```python
from build123d import *

# Parameters (mm, degrees)
CROQUIS1_R              = 100
SALIENTE_EXTRUIR1_DEPTH = 3
CROQUIS3_R              = 110
CORTAR_EXTRUIR1_DEPTH   = 3
REDONDEO1_R             = 10
CORTAR_EXTRUIR2_DEPTH   = 10
CORTAR_EXTRUIR3_DEPTH   = 10
CROQUIS8_R              = 1.5
CROQUIS8_R_2            = 1.502317269
CROQUIS8_R_3            = 2
CORTAR_EXTRUIR4_DEPTH   = 10
CROQUIS9_R              = 1.5
CROQUIS9_W              = 4.5
CROQUIS9_H              = 7.5
CROQUIS9_W_2            = 7.5
CROQUIS9_H_2            = 4.5
CORTAR_EXTRUIR5_DEPTH   = 10


with BuildPart() as part:
    # Croquis1 → Saliente-Extruir1 (new body)
    with BuildSketch(Plane.XY):
        Circle(CROQUIS1_R)
    extrude(amount=SALIENTE_EXTRUIR1_DEPTH)

    # Croquis3 → Cortar-Extruir1 (cut)
    with BuildSketch(Plane.XY.offset(3)):
        with Locations((190, 0)):
            Circle(CROQUIS3_R)
    extrude(amount=-CORTAR_EXTRUIR1_DEPTH, mode=Mode.SUBTRACT)

    # Redondeo1
    redondeo1_edges = [part.edges().sort_by_distance(p)[0] for p in [
        (89.473684211, -44.659375654, 1.5),
        (89.473684211, 44.659375654, 1.5),
    ]]
    fillet(redondeo1_edges, radius=REDONDEO1_R)

    # Croquis5 → Cortar-Extruir2 (cut)
    with BuildSketch(Plane.XY.offset(3)):
        Polygon((-29.69848481, -9.899494937), (-9.899494937, -29.69848481), (-64.346717088, -84.145706961), (-84.145706961, -64.346717088), align=None)
        Polygon((-9.899494937, 29.69848481), (-29.69848481, 9.899494937), (-84.145706961, 64.346717088), (-64.346717088, 84.145706961), align=None)
        Polygon((29.69848481, 9.899494937), (9.899494937, 29.69848481), (64.346717088, 84.145706961), (84.145706961, 64.346717088), align=None)
        Polygon((9.899494937, -29.69848481), (29.69848481, -9.899494937), (84.145706961, -64.346717088), (64.346717088, -84.145706961), align=None)
    extrude(amount=-CORTAR_EXTRUIR2_DEPTH, mode=Mode.SUBTRACT)

    # Croquis7 → Cortar-Extruir3 (cut)
    with BuildSketch(Plane.XY.offset(3)):
        Polygon((-71.939339828, -40.119534675), (-40.119534675, -71.939339828), (-57.090097423, -88.909902577), (-88.909902577, -57.090097423), align=None)
        Polygon((-40.119534675, 71.939339828), (-71.939339828, 40.119534675), (-88.909902577, 57.090097423), (-57.090097423, 88.909902577), align=None)
        Polygon((71.939339828, 40.119534675), (40.119534675, 71.939339828), (57.090097423, 88.909902577), (88.909902577, 57.090097423), align=None)
        Polygon((40.119534675, -71.939339828), (71.939339828, -40.119534675), (88.909902577, -57.090097423), (57.090097423, -88.909902577), align=None)
        Polygon((-21.566756826, -18.03122292), (-18.03122292, -21.566756826), (-14.495689014, -18.03122292), (-18.03122292, -14.495689014), align=None)
        Polygon((-21.566756826, 18.03122292), (-18.03122292, 14.495689014), (-14.495689014, 18.03122292), (-18.03122292, 21.566756826), align=None)
        Polygon((18.03122292, 21.566756826), (14.495689014, 18.03122292), (18.03122292, 14.495689014), (21.566756826, 18.03122292), align=None)
        Polygon((21.566756826, -18.03122292), (18.03122292, -14.495689014), (14.495689014, -18.03122292), (18.03122292, -21.566756826), align=None)
    extrude(amount=-CORTAR_EXTRUIR3_DEPTH, mode=Mode.SUBTRACT)

    # Croquis8 → Cortar-Extruir4 (cut)
    with BuildSketch(Plane.XY.offset(3)):
        with Locations((-64.762205999, 40.904423202)):
            Circle(CROQUIS8_R)
        with Locations((-48.852303422, 24.994520625)):
            Circle(CROQUIS8_R_2)
        with Locations((-24.994520625, 48.852303422)):
            Circle(CROQUIS8_R)
        with Locations((-40.904423202, 64.762205999)):
            Circle(CROQUIS8_R)
        with Locations((64.762205999, 40.904423202)):
            Circle(CROQUIS8_R)
        with Locations((48.852303422, 24.994520625)):
            Circle(CROQUIS8_R)
        with Locations((24.994520625, 48.852303422)):
            Circle(CROQUIS8_R_2)
        with Locations((40.904423202, 64.762205999)):
            Circle(CROQUIS8_R)
        with Locations((40.904423202, -64.762205999)):
            Circle(CROQUIS8_R)
        with Locations((24.994520625, -48.852303422)):
            Circle(CROQUIS8_R)
        with Locations((48.852303422, -24.994520625)):
            Circle(CROQUIS8_R_2)
        with Locations((64.762205999, -40.904423202)):
            Circle(CROQUIS8_R)
        with Locations((-64.762205999, -40.904423202)):
            Circle(CROQUIS8_R)
        with Locations((-48.852303422, -24.994520625)):
            Circle(CROQUIS8_R)
        with Locations((-24.994520625, -48.852303422)):
            Circle(CROQUIS8_R_2)
        with Locations((-40.904423202, -64.762205999)):
            Circle(CROQUIS8_R)
        with Locations((0, 92)):
            Circle(CROQUIS8_R_3)
        with Locations((0, -92)):
            Circle(CROQUIS8_R_3)
        with Locations((72, 31.694913472)):
            Circle(CROQUIS8_R_3)
        with Locations((72, -31.694913472)):
            Circle(CROQUIS8_R_3)
        with Locations((-85, -30)):
            Circle(CROQUIS8_R_3)
        with Locations((-85, 30)):
            Circle(CROQUIS8_R_3)
    extrude(amount=-CORTAR_EXTRUIR4_DEPTH, mode=Mode.SUBTRACT)

    # Croquis9 → Cortar-Extruir5 (cut)
    with BuildSketch(Plane.XY.offset(3)):
        with Locations((73.1, -4.5)):
            Circle(CROQUIS9_R)
        with Locations((35.9, 4.5)):
            Circle(CROQUIS9_R)
        with Locations((73.1, 4.5)):
            Circle(CROQUIS9_R)
        with Locations((35.9, -4.5)):
            Circle(CROQUIS9_R)
        with Locations((-91.190074744, 4.5)):
            Circle(CROQUIS9_R)
        with Locations((-91.190074744, -4.5)):
            Circle(CROQUIS9_R)
        with Locations((-53.990074744, 4.5)):
            Circle(CROQUIS9_R)
        with Locations((-53.990074744, -4.5)):
            Circle(CROQUIS9_R)
        with Locations((-4.5, 85)):
            Circle(CROQUIS9_R)
        with Locations((4.5, 85)):
            Circle(CROQUIS9_R)
        with Locations((-4.5, 47.8)):
            Circle(CROQUIS9_R)
        with Locations((4.5, 47.8)):
            Circle(CROQUIS9_R)
        with Locations((-4.5, -47.8)):
            Circle(CROQUIS9_R)
        with Locations((4.5, -47.8)):
            Circle(CROQUIS9_R)
        with Locations((4.5, -85)):
            Circle(CROQUIS9_R)
        with Locations((-4.5, -85)):
            Circle(CROQUIS9_R)
        with Locations((39.85, 0)):
            Rectangle(CROQUIS9_W, CROQUIS9_H)
        with Locations((0, -51.75)):
            Rectangle(CROQUIS9_W_2, CROQUIS9_H_2)
        with Locations((-57.940074744, 0)):
            Rectangle(CROQUIS9_W, CROQUIS9_H)
        with Locations((0, 51.75)):
            Rectangle(CROQUIS9_W_2, CROQUIS9_H_2)
    extrude(amount=-CORTAR_EXTRUIR5_DEPTH, mode=Mode.SUBTRACT)


solid = part.part
```
The model under review builds one solid part; all positions refer to its coordinate system, in mm. A direction names the side the tool comes from. Round coordinates to 2 decimals unless told otherwise and drop trailing zeros. Order: outer loops, then holes, each group sorted by start corner. A loop starts at its lowest first (then second) coordinate and runs counter-clockwise, first axis right, second up. Notation, with made-up numbers: (-2, -37.75) - (5, -37.75) arc R11 cw to (5, -24.75) - close; hole circle Ø10 at (78.5, -2.5). An arc over 180 degrees is marked (long way). Answer in a Markdown table with one row per item.
(1) Machinability: for faces 5 (the face through (-68.89, 43.17, 1.52)), 6 (the face through (-43.08, 68.98, 1.52)), 7 (the face through (25.7, 13.9, 1.5)), 8 (the face through (78.28, -46.46, 1.52)), which of the approach directions +Z, -Z, +X, -X, +Y, -Y give a long, thin tool a straight path to every point of the face, cutting with its end or side? Answer none if there is none.
Result set:
| item | result |
|---|---|
| face 5 | +Z, -Z, +Y |
| face 6 | +Z, -Z, -X |
| face 7 | +Z, -Z |
| face 8 | +Z, -Z, -Y |
(2) Take a section at A-A on z = 1.5. Count the separate pieces of the cut face and the enclosed holes in it, plus the area to 3 significant figures.
Result set:
| item | result |
|---|---|
| separate pieces | 1 |
| enclosed holes | 42 |
| area | 20,300 mm2 |
(3) Take a section at B-B on y = -58.5. Write out the cut boundary in (x, z).
Result set:
| item | result |
|---|---|
| outline | (-38.7, 0) - (38.7, 0) - (38.7, 3) - (-38.7, 3) - close |
(4) For line 1 (Y direction, x = 17, z = 0.35); line 2 (Y direction, x = -12.5, z = 2.65); line 3 (Y direction, x = 27, z = 1.25), list the stretches that pass through material, from the lowest coordinate up. Write a range as from..to.
Result set:
| item | result |
|---|---|
| line 1 | y = -98.54..-36.8, -22.6..-20.54, -15.53..15.53, 20.54..22.6, 36.8..98.54 |
| line 2 | y = -99.22..-32.3, -27.1..27.1, 32.3..99.22 |
| line 3 | y = -96.29..-46.8, -12.6..12.6, 46.8..96.29 |
(5) Clearance check with flat-ended pins moving along their axes: P1, Ø1.5, axis at x = -23.5, z = 1.5, coming from the -Y side; P2, Ø5, axis at x = -85, y = -30, coming from the +Z side; P3, Ø1.5, axis at y = -50.5, z = 1, coming from the +X side. State where each tip first meets the part, or that it passes through.
Result set:
| item | result |
|---|---|
| P1 | stops at y = -97.38 |
| P2 | stops at z = 3 |
| P3 | stops at x = 86.75 |
(6) Mouldability with a two-part tool opening along Y and no side actions: class faces 1 (the face through (43.08, -68.98, 1.52)), 2 (the face through (-7, 1, 0)), 3 (the face through (47.6, -27.8, 1.5)), 4 (the face through (0.782, 99.997, 1.479)) as released by +Y, released by -Y, zero draft, split by the parting line, or undercut.
Result set:
| item | result |
|---|---|
| face 1 | undercut |
| face 2 | zero draft |
| face 3 | undercut |
| face 4 | released by +Y |
